```python
from build123d import *

# Parameters (mm, degrees)
BODY_DEPTH           = 4.75
M5_CLEARANCE_HOLE1_D = 5.5


with BuildPart() as part:
    # Sketch1 → Body (new, symmetric)
    with BuildSketch(Plane(origin=(0, 0, 0), x_dir=(0, 0, -1), z_dir=(1, 0, 0))):
        Polygon((-3.5, 0), (3.5, 0), (4.75, 1.3), (4.75, 3.3), (3, 3.3), (3, 4.3), (-3, 4.3), (-3, 3.3), (-4.75, 3.3), (-4.75, 1.3), align=None)
    extrude(amount=BODY_DEPTH, both=True)

    # M5 Clearance Hole1 (through all)
    with Locations(Plane(origin=(0, 4.3, 0), x_dir=(1, 0, 0), z_dir=(0, 1, 0))):
        with Locations((0, 0)):
            Hole(M5_CLEARANCE_HOLE1_D / 2)


solid = part.part
```
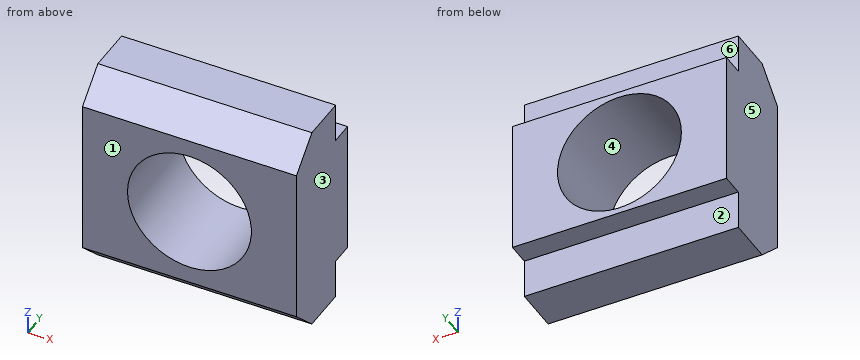
Geometry: final body of the model. Coordinates: model frame, mm. Face numbers are marked on the shaded views. A direction names the side the tool comes from. Give positions to 0.01 mm unless a question says otherwise; leave off trailing zeros. Write each loop counter-clockwise with the first axis right and the second up, starting at its lowest first coordinate (ties: lowest second). Pieces come first, ordered by that corner, then holes.
1. Section query D-D, the plane x = 2.5. Return loops of the section in (y, z), then the cut area to 3 significant figures.
2. Section query A-A, the plane x = 0. Return loops of the section in (y, z).
3. Draft query along X for the marked faces 3, 4, 5 and 6. Return one class per face: released by +X, released by -X, zero draft, split by the parting line, or undercut.
4. Line query: probe 1 along Z at (x, y) = (0, 1.95); probe 2 along X at (y, z) = (0.25, 2); probe 3 along Z at (x, y) = (0, 3.45). Output: solid intervals per line, ascending.
5. Section query C-C, the plane y = 3.65. Return loops of the section in (x, z).
6. Section query B-B, the plane z = 0. Return loops of the section in (x, y), then the cut area to 3 significant figures.
7. Pin query (flat end, axial travel): P1, Ø0.5, axis at x = -1.5, z = 4, coming from the +Y side; P2, Ø0.8, axis at x = -0.5, y = 4, coming from the +Z side; P3, Ø2, axis at x = -1, z = 0, coming from the +Y side; P4, Ø0.5, axis at x = 0.5, y = 4, coming from the -Z side. Return the tip coordinate at first contact, or that it passes through.
8. Reachability of the marked faces 1 and 2 from +Z, -Z, +X, -X, +Y, -Y: full face, straight path, thin tool, end or side. Return the list, or none.
Computed:
1. outline: (0, -3.5) - (1.3, -4.75) - (3.3, -4.75) - (3.3, -3) - (4.3, -3) - (4.3, -1.15) - (0, -1.15) - close; (0, 1.15) - (4.3, 1.15) - (4.3, 3) - (3.3, 3) - (3.3, 4.75) - (1.3, 4.75) - (0, 3.5) - close
1. area: 25.9 mm2
2. outline: (0, -3.5) - (1.3, -4.75) - (3.3, -4.75) - (3.3, -3) - (4.3, -3) - (4.3, -2.75) - (0, -2.75) - close; (0, 2.75) - (4.3, 2.75) - (4.3, 3) - (3.3, 3) - (3.3, 4.75) - (1.3, 4.75) - (0, 3.5) - close
3. face 3: released by +X
3. face 4: undercut
3. face 5: released by -X
3. face 6: zero draft
4. probe 1: z = -4.75 to -2.75, 2.75 to 4.75
4. probe 2: x = -4.75 to -1.89, 1.89 to 4.75
4. probe 3: z = -3 to -2.75, 2.75 to 3
5. outline: (-4.75, -3) - (4.75, -3) - (4.75, 3) - (-4.75, 3) - close; hole circle Ø5.5 at (0, 0)
6. outline: (-4.75, 0) - (-2.75, 0) - (-2.75, 4.3) - (-4.75, 4.3) - close; (2.75, 0) - (4.75, 0) - (4.75, 4.3) - (2.75, 4.3) - close
6. area: 17.2 mm2
7. P1: stops at y = 3.3
7. P2: stops at z = 3
7. P3: passes through
7. P4: stops at z = -3
8. face 1: +Z, -Z, +X, -X, -Y
8. face 2: -Z, +X, -X, +Y
